Geometry check sheet. Reference: the model listing, model coordinates, mm. Face numbers are marked on the shaded views. A direction names the side the tool comes from. Round coordinates to 2 decimals unless told otherwise and drop trailing zeros. Order: outer loops, then holes, each group sorted by start corner. A loop starts at its lowest first (then second) coordinate and runs counter-clockwise, first axis right, second up.
(1) Set-up check for the marked faces 4, 5 and 6: record each of +Z, -Z, +X, -X, +Y, -Y from which the full face is reachable in a straight line by a thin tool's end or side.
(2) Sectioned sample at A-A (z = -19.4). Record the boundary of the cut face in (x, y).
(3) Release check for a two-part mould opening along X. For the marked faces 1, 2 and 3 record: +X half, -X half, draft (parallel to the pull), parting line (faces both ways), or undercut.
(4) Sectioned sample at B-B (y = -12.75). Give the number of separate pieces and of enclosed holes in the cut face, plus the area to 3 significant figures.
(5) Material ranges on line 1 along Y through (x, z) = (6.75, 15); line 2 along Y through (x, z) = (7.25, 15); line 3 along Y through (x, z) = (11.75, 24.5), recorded low to high.
(6) Sectioned sample at D-D (z = -1.5). Record the boundary of the cut face in (x, y), plus the area to 3 significant figures.
(7) Go/stop test with flat-tipped pins: pin 1 (2 mm diameter, centred on y = -9.5, z = -11.5, fed in from -X); pin 2 (5 mm diameter, centred on x = 10, y = 13, fed in from -Z) (3 decimals); pin 3 (4 mm diameter, centred on x = 4.5, z = 7, fed in from -Y); pin 4 (1 mm diameter, centred on x = 17, z = 19.5, fed in from -Y). Record where each tip stops, or that it passes through.
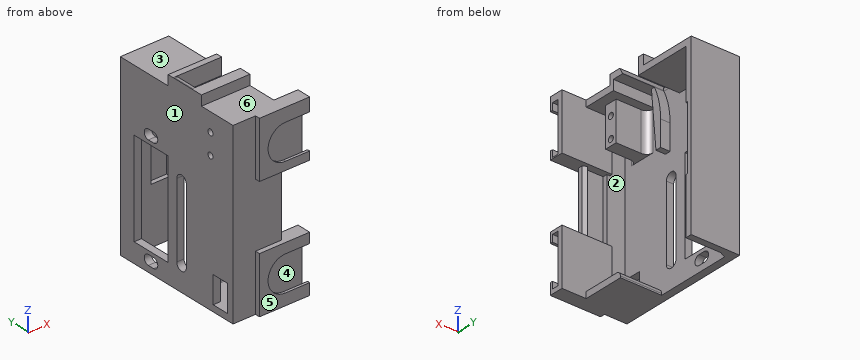
from build123d import *

# Parameters (mm, degrees)
MAIN_EXTRUDE_DEPTH            = 2.2875
WALLS_START                   = 2.2875
WALLS_DEPTH                   = 13
CORNER_SUPPORT_DEPTH          = 2
SKETCH2_R                     = 0.95
SKETCH2_W                     = 2.4
SKETCH2_H                     = 4
SKETCH2_W_2                   = 1
SWITCH_SPACER_DEPTH           = 9.9
ARM_SUPPORT_EXTRUDE_DEPTH     = 3
ARM_SUPPORT_CURVE_DEPTH       = 40.380356778
FILLET4_R                     = 2
FILLET3_R                     = 2
SKETCH2_5_R                   = 0.95
SWITCH_MOUNT_HOLES_DEPTH      = 40.380356889
SWITCH_MOUNT_HOLES_DEPTH_BACK = 40.380356889
SKETCH4_W                     = 8.5
SKETCH4_H                     = 5.5
WIRE_HOLE_DEPTH               = 40.380356889
SKETCH25_W                    = 6
SKETCH25_H                    = 1.35
FEMALE_SNAP_DEPTH             = 10.125
SKETCH5_W                     = 30
SKETCH5_H                     = 12.75
SERVO_HOLE_DEPTH              = 40.380356889
SKETCH30_W                    = 15.7875
SKETCH30_H                    = 0.9
SKETCH30_W_2                  = 17.7875
SKETCH30_H_2                  = 1.5
MAGNET_EXTRUDE_1_DEPTH        = 7.625
MAGNET_EXTRUDE_1_DEPTH_BACK   = 8.2
SKETCH29_R                    = 7.7
MAGNET_HOLE_DEPTH             = 2.1
SKETCH31_R                    = 5.5
MAGNET_THRU_HOLE_DEPTH        = 58.632218961


with BuildPart() as part:
    # Sketch1 → Main Extrude (new body)
    with BuildSketch(Plane(origin=(0, 0, 0), x_dir=(0, 0, -1), z_dir=(1, 0, 0))):
        Polygon((-30.5, -9.35), (-27.325, -9.35), (-27.325, -21.25), (28.5, -21.25), (28.5, 21.25), (-27.325, 21.25), (-27.325, 3.2), (-30.5, 3.2), align=None)
        with BuildLine():
            Line((20.7, -3.65), (-2.8, -3.65))
            ThreePointArc((-2.8, -3.65), (-4.6, -1.85), (-2.8, -0.05))
            Line((-2.8, -0.05), (20.7, -0.05))
            ThreePointArc((20.7, -0.05), (22.5, -1.85), (20.7, -3.65))
        make_face(mode=Mode.SUBTRACT)
    extrude(amount=MAIN_EXTRUDE_DEPTH)

    # Sketch1_3 → Walls (add)
    with BuildSketch(Plane(origin=(0, 0, 0), x_dir=(0, 0, -1), z_dir=(1, 0, 0)).offset(WALLS_START)):
        Polygon((-25.325, 19.25), (28.5, 19.25), (28.5, 21.25), (-27.325, 21.25), (-27.325, 3.2), (-30.5, 3.2), (-30.5, 1.3), (-25.325, 1.3), align=None)
        with BuildLine():
            Line((28.5, -5.425), (28, -5.425))
            ThreePointArc((28, -5.425), (26.939339828, -5.864339828), (26.5, -6.925))
            Line((26.5, -6.925), (26.5, -19.25))
            Line((26.5, -19.25), (-25.325, -19.25))
            Line((-25.325, -19.25), (-25.325, -8.1))
            Line((-25.325, -8.1), (-28.5, -8.1))
            Line((-28.5, -8.1), (-28.5, -4.45))
            Line((-28.5, -4.45), (-30.5, -4.45))
            Line((-30.5, -4.45), (-30.5, -9.35))
            Line((-30.5, -9.35), (-27.325, -9.35))
            Line((-27.325, -9.35), (-27.325, -21.25))
            Line((-27.325, -21.25), (28.5, -21.25))
            Line((28.5, -21.25), (28.5, -5.425))
        make_face()
    extrude(amount=WALLS_DEPTH)

    # Sketch22 → Corner Support (add)
    with BuildSketch(Plane(origin=(0, 0, -28.5), x_dir=(-1, 0, 0), z_dir=(0, 0, -1))):
        Polygon((-4.2875, 19.25), (-2.2875, 18.25), (-2.2875, 19.25), align=None)
    extrude(amount=-CORNER_SUPPORT_DEPTH)

    # Sketch2 → Switch Spacer (add)
    with BuildSketch(Plane(origin=(2.2875, 0, 0), x_dir=(0, 0, -1), z_dir=(1, 0, 0))):
        Polygon((-14.05, -10.75), (-17.05, -10.75), (-17.05, -14.75), (-14.05, -14.75), (-14.05, -12.75), align=None)
        with Locations((-15, -12.75)):
            Circle(SKETCH2_R, mode=Mode.SUBTRACT)
        with Locations((-15, -12.75)):
            Circle(SKETCH2_R)
        Polygon((-19.45, -10.75), (-22.45, -10.75), (-22.45, -12.75), (-22.45, -14.75), (-19.45, -14.75), align=None)
        with BuildLine():
            ThreePointArc((-20.55, -12.75), (-21.5, -13.7), (-22.45, -12.75))
            ThreePointArc((-22.45, -12.75), (-21.5, -11.8), (-20.55, -12.75))
        make_face(mode=Mode.SUBTRACT)
        with Locations((-21.5, -12.75)):
            Circle(SKETCH2_R)
        Polygon((-22.45, -12.75), (-22.45, -10.75), (-25.325, -10.75), (-25.325, -14.75), (-22.45, -14.75), align=None)
        with Locations((-18.25, -12.75)):
            Rectangle(SKETCH2_W, SKETCH2_H)
        with Locations((-13.55, -12.75)):
            Rectangle(SKETCH2_W_2, SKETCH2_H)
    extrude(amount=SWITCH_SPACER_DEPTH)

    # Sketch3 → Arm Support Extrude (add)
    with BuildSketch(Plane(origin=(2.2875, 0, 0), x_dir=(0, 0, -1), z_dir=(1, 0, 0))):
        with BuildLine():
            Line((-18.5, -2.25), (-10.5, -2.25))
            Line((-10.5, -2.25), (-10.5, -4))
            Line((-10.5, -4), (-28.5, -5.7))
            Line((-28.5, -5.7), (-30.5, -5.7))
            ThreePointArc((-30.5, -5.7), (-24.743046131, -3.129622151), (-18.5, -2.25))
        make_face()
    extrude(amount=ARM_SUPPORT_EXTRUDE_DEPTH)

    # Sketch7 → Arm Support Curve (cut, through all)
    with BuildSketch(Plane(origin=(2.2875, 0, 0), x_dir=(0, 0, -1), z_dir=(1, 0, 0))):
        with BuildLine():
            Line((-28.5, -4.583410824), (-28.5, -4.45))
            Line((-28.5, -4.45), (-30.5, -4.45))
            Line((-30.5, -4.45), (-30.5, -5.7))
            ThreePointArc((-30.5, -5.7), (-29.627655409, -5.180138898), (-28.73283292, -4.7))
            ThreePointArc((-28.73283292, -4.7), (-28.616584416, -4.641369997), (-28.5, -4.583410824))
        make_face()
    extrude(amount=ARM_SUPPORT_CURVE_DEPTH, mode=Mode.SUBTRACT)

    # Fillet4
    fillet4_edges = [part.edges().sort_by_distance(p)[0] for p in [
        (2.2875, -2.2, 30.5),
    ]]
    fillet(fillet4_edges, radius=FILLET4_R)

    # Fillet3
    fillet3_edges = [part.edges().sort_by_distance(p)[0] for p in [
        (2.2875, -14.75, 19.1875),
        (2.2875, -10.75, 19.1875),
    ]]
    fillet(fillet3_edges, radius=FILLET3_R)

    # Sketch2_5 → Switch Mount Holes (cut, two sides)
    with BuildSketch(Plane(origin=(2.2875, 0, 0), x_dir=(0, 0, -1), z_dir=(1, 0, 0))) as switch_mount_holes_sk:
        with Locations((-21.5, -12.75)):
            Circle(SKETCH2_5_R)
        with Locations((-15, -12.75)):
            Circle(SKETCH2_5_R)
    extrude(amount=SWITCH_MOUNT_HOLES_DEPTH, mode=Mode.SUBTRACT)
    extrude(switch_mount_holes_sk.sketch, amount=-SWITCH_MOUNT_HOLES_DEPTH_BACK, mode=Mode.SUBTRACT)

    # Sketch4 → Wire Hole (cut, through all)
    with BuildSketch(Plane(origin=(2.2875, 0, 0), x_dir=(0, 0, -1), z_dir=(1, 0, 0))):
        with Locations((22.25, -16.5)):
            Rectangle(SKETCH4_W, SKETCH4_H)
    extrude(amount=-WIRE_HOLE_DEPTH, mode=Mode.SUBTRACT)

    # Sketch25 → Female Snap (cut, symmetric)
    with BuildSketch(Plane(origin=(0, 0, -0.5875), x_dir=(-1, 0, 0), z_dir=(0, 0, -1))):
        with Locations((-11.0375, -19.925)):
            Rectangle(SKETCH25_W, SKETCH25_H)
        Polygon((-15.2875, -19.25), (-15.2875, -19.91463679), (-14.0375, -19.25), align=None)
        with Locations((-11.0375, 19.925)):
            Rectangle(SKETCH25_W, SKETCH25_H)
        Polygon((-15.2875, 19.91463679), (-15.2875, 19.25), (-14.0375, 19.25), align=None)
    extrude(amount=FEMALE_SNAP_DEPTH, both=True, mode=Mode.SUBTRACT)

    # Sketch5 → Servo Hole (cut, through all)
    with BuildSketch(Plane(origin=(2.2875, 0, 0), x_dir=(0, 0, -1), z_dir=(1, 0, 0))):
        with Locations((7.35, 9.675)):
            Rectangle(SKETCH5_W, SKETCH5_H)
        with BuildLine():
            Line((-8.75, 10.675), (-8.75, 8.675))
            ThreePointArc((-8.75, 8.675), (-10.3, 7.125), (-11.85, 8.675))
            Line((-11.85, 8.675), (-11.85, 10.675))
            ThreePointArc((-11.85, 10.675), (-10.3, 12.225), (-8.75, 10.675))
        make_face()
        with BuildLine():
            Line((26.55, 10.675), (26.55, 8.675))
            ThreePointArc((26.55, 8.675), (25, 7.125), (23.45, 8.675))
            Line((23.45, 8.675), (23.45, 10.675))
            ThreePointArc((23.45, 10.675), (25, 12.225), (26.55, 10.675))
        make_face()
    extrude(amount=-SERVO_HOLE_DEPTH, mode=Mode.SUBTRACT)

    # Sketch30 → Magnet Extrude 1 (add, two sides)
    with BuildSketch(Plane(origin=(15.2875, 0, 0), x_dir=(0, 0, -1), z_dir=(1, 0, 0))) as magnet_extrude_1_sk:
        Polygon((-27.325, -18.35), (-27.325, -21.25), (-9.5375, -21.25), (-9.5375, -19.91463679), (-9.5375, -19.25), (-25.325, -19.25), (-25.325, -18.35), align=None)
        with Locations((-17.43125, -18.8)):
            Rectangle(SKETCH30_W, SKETCH30_H)
        with Locations((19.60625, -22)):
            Rectangle(SKETCH30_W_2, SKETCH30_H_2)
        Polygon((10.7125, -19.91463679), (10.7125, -21.25), (28.5, -21.25), (28.5, -18.35), (26.5, -18.35), (26.5, -19.25), (10.7125, -19.25), align=None)
        with Locations((-18.43125, -22)):
            Rectangle(SKETCH30_W_2, SKETCH30_H_2)
        with Locations((18.60625, -18.8)):
            Rectangle(SKETCH30_W, SKETCH30_H)
    extrude(amount=MAGNET_EXTRUDE_1_DEPTH)
    extrude(magnet_extrude_1_sk.sketch, amount=-MAGNET_EXTRUDE_1_DEPTH_BACK)

    # Sketch29 → Magnet Hole (cut)
    with BuildSketch(Plane(origin=(0, -21.95, 0), x_dir=(1, 0, 0), z_dir=(0, 1, 0))):
        with Locations((15.2875, -17.625)):
            Circle(SKETCH29_R)
        with BuildLine():
            ThreePointArc((22.9125, -18.697089082), (20.338980677, -23.436414885), (15.2875, -25.325))
            Line((15.2875, -25.325), (22.9125, -25.325))
            Line((22.9125, -25.325), (22.9125, -18.697089082))
        make_face()
        with BuildLine():
            Line((22.9125, -9.925), (15.2875, -9.925))
            ThreePointArc((15.2875, -9.925), (20.338980677, -11.813585115), (22.9125, -16.552910918))
            Line((22.9125, -16.552910918), (22.9125, -9.925))
        make_face()
        with Locations((15.2875, 19.4)):
            Circle(SKETCH29_R)
        with BuildLine():
            ThreePointArc((22.9125, 18.327910918), (20.338980677, 13.588585115), (15.2875, 11.7))
            Line((15.2875, 11.7), (22.9125, 11.7))
            Line((22.9125, 11.7), (22.9125, 18.327910918))
        make_face()
        with BuildLine():
            Line((22.9125, 27.1), (15.2875, 27.1))
            ThreePointArc((15.2875, 27.1), (20.338980677, 25.211414885), (22.9125, 20.472089082))
            Line((22.9125, 20.472089082), (22.9125, 27.1))
        make_face()
        with BuildLine():
            ThreePointArc((22.9875, -17.625), (22.968727116, -17.087645368), (22.9125, -16.552910918))
            Line((22.9125, -16.552910918), (22.9125, -18.697089082))
            ThreePointArc((22.9125, -18.697089082), (22.968727116, -18.162354632), (22.9875, -17.625))
        make_face()
        with BuildLine():
            Line((22.9125, 20.472089082), (22.9125, 18.327910918))
            ThreePointArc((22.9125, 18.327910918), (22.968727116, 18.862645368), (22.9875, 19.4))
            ThreePointArc((22.9875, 19.4), (22.968727116, 19.937354632), (22.9125, 20.472089082))
        make_face()
    extrude(amount=MAGNET_HOLE_DEPTH, mode=Mode.SUBTRACT)

    # Sketch31 → Magnet Thru Hole (cut, through all)
    with BuildSketch(Plane.XZ.offset(21.95)):
        with Locations((15.2875, 17.625)):
            Circle(SKETCH31_R)
        with BuildLine():
            Line((22.9125, 23.125), (15.2875, 23.125))
            ThreePointArc((15.2875, 23.125), (19.176587297, 21.514087297), (20.7875, 17.625))
            ThreePointArc((20.7875, 17.625), (19.176587297, 13.735912703), (15.2875, 12.125))
            Line((15.2875, 12.125), (22.9125, 12.125))
            Line((22.9125, 12.125), (22.9125, 23.125))
        make_face()
        with Locations((15.2875, -19.4)):
            Circle(SKETCH31_R)
        with BuildLine():
            Line((22.9125, -13.9), (15.2875, -13.9))
            ThreePointArc((15.2875, -13.9), (19.176587297, -15.510912703), (20.7875, -19.4))
            ThreePointArc((20.7875, -19.4), (19.176587297, -23.289087297), (15.2875, -24.9))
            Line((15.2875, -24.9), (22.9125, -24.9))
            Line((22.9125, -24.9), (22.9125, -13.9))
        make_face()
    extrude(amount=MAGNET_THRU_HOLE_DEPTH, mode=Mode.SUBTRACT)


solid = part.part
Answer below:
1. face 4: +X
1. face 5: +Z, -Z, +X, -X, -Y
1. face 6: +Z, +X, -X, -Y
2. outline: (0, -21.25) - (7.09, -21.25) - (7.09, -22.75) - (9.79, -22.75) - (9.79, -21.95) - (7.59, -21.95) - (7.59, -19.85) - (22.91, -19.85) - (22.91, -18.35) - (7.09, -18.35) - (7.09, -19.25) - (0, -19.25) - close; (0, -13.75) - (2.29, -13.75) - (2.29, -3.65) - (0, -3.65) - close; (0, -0.05) - (2.29, -0.05) - (2.29, 3.3) - (0, 3.3) - close; (0, 16.05) - (2.29, 16.05) - (2.29, 19.25) - (15.29, 19.25) - (15.29, 21.25) - (0, 21.25) - close
3. face 1: -X half
3. face 2: undercut
3. face 3: draft
4. separate pieces: 3
4. enclosed holes: 0
4. area: 255 mm2
5. line 1: y = -21.25 to -19.25, -14.75 to -13.7, -11.8 to -10.75, 19.25 to 21.25
5. line 2: y = -22.75 to -18.35, -14.75 to -13.7, -11.8 to -10.75, 19.25 to 21.25
5. line 3: y = -22.75 to -18.35, -14.75 to -10.75, 19.25 to 21.25
6. outline: (0, -21.25) - (15.29, -21.25) - (15.29, -19.91) - (14.04, -19.25) - (14.04, -20.6) - (8.04, -20.6) - (8.04, -19.25) - (2.29, -19.25) - (2.29, -3.65) - (0, -3.65) - close; (0, -0.05) - (2.29, -0.05) - (2.29, 3.3) - (0, 3.3) - close; (0, 16.05) - (2.29, 16.05) - (2.29, 19.25) - (8.04, 19.25) - (8.04, 20.6) - (14.04, 20.6) - (14.04, 19.25) - (15.29, 19.91) - (15.29, 21.25) - (0, 21.25) - close
6. area: 94.8 mm2
7. pin 1: stops at x = 0
7. pin 2: stops at z = 25.325
7. pin 3: stops at y = -21.25
7. pin 4: stops at y = -19.85
